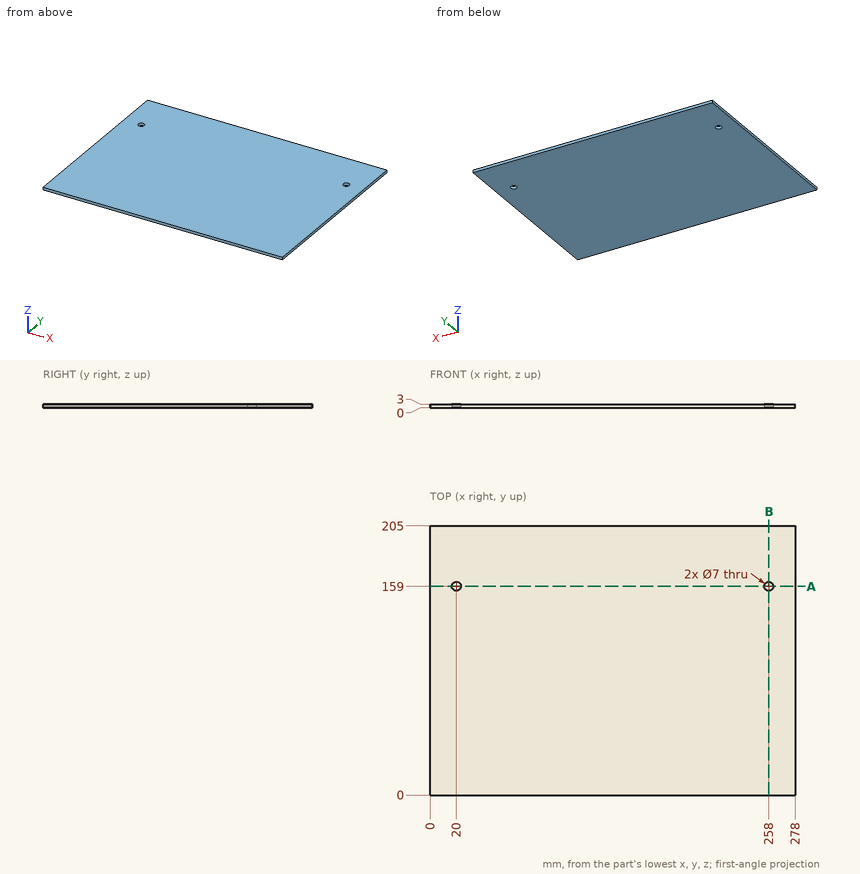
Part print with two shaded views. Sizes in mm from the minimum x, y, z corner. Coordinates: 2 decimals unless noted, no trailing zeros. Write each loop counter-clockwise with the first axis right and the second up, starting at its lowest first coordinate (ties: lowest second). Pieces come first, ordered by that corner, then holes. Notation, with made-up numbers: M -11,45 L 25,45 A26 ccw 25,76 Z; hole C -38.5,-23.75 d1. An arc over 180 degrees is marked long. Return JSON: item names as keys, results as strings.
Item 1: Slice it at B-B, the plane x = 258. Write the cut outline in (y, z).
Findings below:
{"outline": "M 0,0 L 155.5,0 L 155.5,3 L 0,3 Z; M 162.5,0 L 205,0 L 205,3 L 162.5,3 Z"}
Item 2: Slice it at A-A, the plane y = 159. Write the cut outline in (x, z).
Findings below:
{"outline": "M 0,0 L 16.5,0 L 16.5,3 L 0,3 Z; M 23.5,0 L 254.5,0 L 254.5,3 L 23.5,3 Z; M 261.5,0 L 278,0 L 278,3 L 261.5,3 Z"}
Item 3: Drop a flat-ended pin along its axis: pin 1 Ø5.5 at (x, y) = (20, 159) entering from -Z. Give the stop position or say it passes through.
Findings below:
{"pin 1": "passes through"}
Item 4: Probe line 1 (X direction, y = 159, z = 2.35); line 2 (Y direction, x = 20, z = 1.95). List the from-to ranges inside material, lowest first. Write a range as from..to.
Findings below:
{"line 1": "x = 0..16.5, 23.5..254.5, 261.5..278", "line 2": "y = 0..155.5, 162.5..205"}
